The drawing under review shows one solid part. Ordinate dimensions are in mm from its lowest x, y, z. A direction names the side the tool comes from. Round coordinates to 2 decimals unless told otherwise and drop trailing zeros. Loops run counter-clockwise (first coordinate to the right, second up) from the corner with the lowest first, then second, coordinate; pieces in that order, holes last. Notation, with made-up numbers: (-25.5, 70) -> (23.5, 70) arc R27 ccw to (23.5, 100) -> close; hole circle Ø9 at (67.25, -26.5). An arc over 180 degrees is marked (long way). Use a Markdown table: item, result. Add a question column.
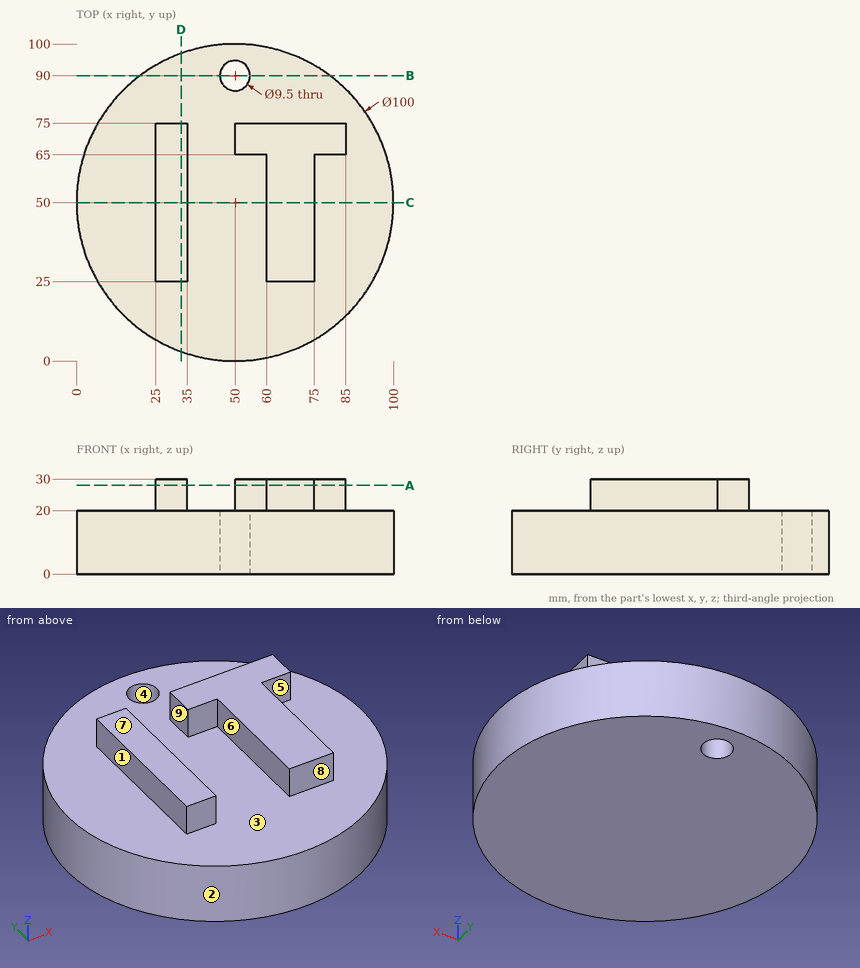
1. Mouldability with a two-part tool opening along X and no side actions: class the marked faces 1, 2, 3 and 4 as +X half, -X half, draft (parallel to the pull), parting line (faces both ways), or undercut.
2. For the marked faces 5, 6, 7, 8 and 9, list the 3-axis set-ups (+Z, -Z, +X, -X, +Y, -Y) from which the entire face can be reached by the end or side of a thin tool; tool diameter is ignored.
3. Insertion check: P1, Ø3, axis at y = 45, z = 26, coming from the +X side; P2, Ø5, axis at x = 66.5, z = 23.5, coming from the -Y side; P3, Ø10, axis at y = 72.5, z = 10.5, coming from the -X side. Each pin has a flat end and moves straight along its axis. Give the tip position at first contact, or say it passes through.
4. Consider section A-A on z = 28. State the section outline as (x, y) points.
5. Consider section C-C on y = 50. State the section outline as (x, z) points.
6. Consider section B-B on y = 90. State the section outline as (x, z) points, plus the area to 3 significant figures.
7. To check wall thickness, follow probe 1 along Y at (x, z) = (50, 7); probe 2 along Z at (x, y) = (12, 39); probe 3 along Y at (x, z) = (32, 21.25). State the ranges of each line that lie inside material, in increasing order. Write a range as from..to.
8. Consider section D-D on x = 33. State the section outline as (y, z) points.
Verdict:
| question | item | result |
|---|---|---|
| 1 | face 1 | -X half |
| 1 | face 2 | parting line |
| 1 | face 3 | undercut |
| 1 | face 4 | undercut |
| 2 | face 5 | +Z, +X, -Y |
| 2 | face 6 | +Z, -Y |
| 2 | face 7 | +Z, +X, -X, +Y, -Y |
| 2 | face 8 | +Z, +X, -X, -Y |
| 2 | face 9 | +Z, +Y, -Y |
| 3 | P1 | stops at x = 75 |
| 3 | P2 | stops at y = 25 |
| 3 | P3 | stops at x = 3.16 |
| 4 | outline | (25, 25) -> (35, 25) -> (35, 75) -> (25, 75) -> close; (50, 65) -> (60, 65) -> (60, 25) -> (75, 25) -> (75, 65) -> (85, 65) -> (85, 75) -> (50, 75) -> close |
| 5 | outline | (0, 0) -> (100, 0) -> (100, 20) -> (75, 20) -> (75, 30) -> (60, 30) -> (60, 20) -> (35, 20) -> (35, 30) -> (25, 30) -> (25, 20) -> (0, 20) -> close |
| 6 | outline | (20, 0) -> (45.25, 0) -> (45.25, 20) -> (20, 20) -> close; (54.75, 0) -> (80, 0) -> (80, 20) -> (54.75, 20) -> close |
| 6 | area | 1,010 mm² |
| 7 | probe 1 | y = 0..85.25, 94.75..100 |
| 7 | probe 2 | z = 0..20 |
| 7 | probe 3 | y = 25..75 |
| 8 | outline | (2.98, 0) -> (97.02, 0) -> (97.02, 20) -> (75, 20) -> (75, 30) -> (25, 30) -> (25, 20) -> (2.98, 20) -> close |
